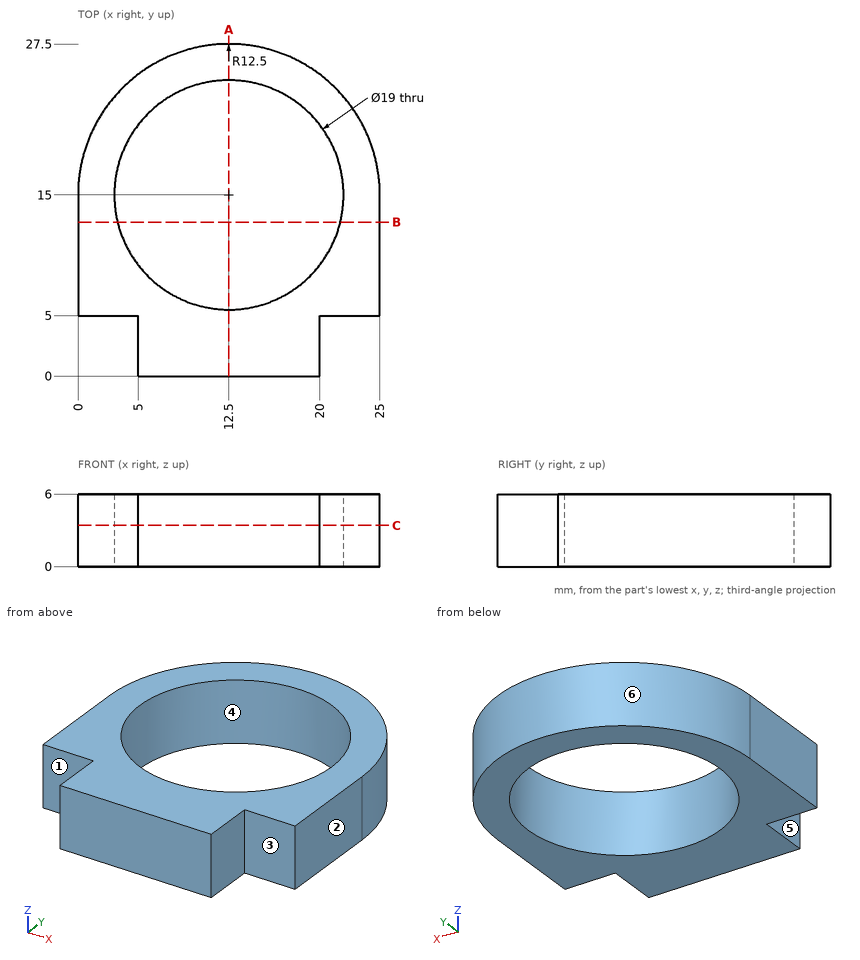
Part print with two shaded views. Sizes in mm from the minimum x, y, z corner. A direction names the side the tool comes from. Coordinates: 2 decimals unless noted, no trailing zeros. Order: outer loops, then holes, each group sorted by start corner. A loop starts at its lowest first (then second) coordinate and runs counter-clockwise, first axis right, second up. Notation, with made-up numbers: M 53.5,-30.75 L 59.5,-30.75 A28 ccw 59.5,5.25 Z; hole C 38.5,75.5 d1. An arc over 180 degrees is marked long. Use a Markdown table: item, result.
(1) Probe L1, parallel to Y at x = 12.25, z = 3.5; L2, parallel to Y at x = 7.5, z = 0.6; L3, parallel to X at y = 11, z = 2.4. List the from-to ranges inside material, lowest first.
A:
| item | result |
|---|---|
| L1 | y = 0 to 5.5, 24.5 to 27.5 |
| L2 | y = 0 to 6.92, 23.08 to 26.46 |
| L3 | x = 0 to 3.88, 21.12 to 25 |
(2) Flat gauge pins, fed straight in: pin 1 (12 mm diameter, centred on x = 20.5, y = 9.5, fed in from -Z); pin 2 (2.5 mm diameter, centred on y = 3.5, z = 3, fed in from +X). Where does each tip first touch, or does it go through?
A:
| item | result |
|---|---|
| pin 1 | stops at z = 0 |
| pin 2 | stops at x = 20 |
(3) Cut at C-C on z = 3.4. Write the cut outline in (x, y), then the cut area to 3 significant figures.
A:
| item | result |
|---|---|
| outline | M 0,5 L 5,5 L 5,0 L 20,0 L 20,5 L 25,5 L 25,15 A12.5 ccw 0,15 Z; hole C 12.5,15 d19 |
| area | 287 mm^2 |
(4) Cut at B-B on y = 12.75. Write the cut outline in (x, z), then the cut area to 3 significant figures.
A:
| item | result |
|---|---|
| outline | M 0,0 L 3.27,0 L 3.27,6 L 0,6 Z; M 21.73,0 L 25,0 L 25,6 L 21.73,6 Z |
| area | 39.2 mm^2 |
(5) Cut at A-A on x = 12.5. Write the cut outline in (y, z), then the cut area to 3 significant figures.
A:
| item | result |
|---|---|
| outline | M 0,0 L 5.5,0 L 5.5,6 L 0,6 Z; M 24.5,0 L 27.5,0 L 27.5,6 L 24.5,6 Z |
| area | 51.0 mm^2 |
(6) Pull direction Y, two halves, no side cores. Call the marked faces 4, 5 and 6: released by +Y, released by -Y, zero draft, split by the parting line, or undercut.
A:
| item | result |
|---|---|
| face 4 | undercut |
| face 5 | zero draft |
| face 6 | released by +Y |
(7) Tool access for the marked faces 1, 2 and 3: list every direction of +Z, -Z, +X, -X, +Y, -Y with a clear straight run to the whole face (end or side of a thin tool).
A:
| item | result |
|---|---|
| face 1 | +Z, -Z, -X, -Y |
| face 2 | +Z, -Z, +X, +Y, -Y |
| face 3 | +Z, -Z, +X, -Y |
